Check sheet for the modelled part. Datum: model origin and axes. Units: mm. A direction names the side the tool comes from. Round coordinates to 2 decimals unless told otherwise and drop trailing zeros. Order: outer loops, then holes, each group sorted by start corner. A loop starts at its lowest first (then second) coordinate and runs counter-clockwise, first axis right, second up.
Q1. Cross-section at A-A on z = 25. Record the cut outline in (x, y).
Q2. Mould release check, pull along X, two halves, no side actions. Record for faces 1 (the flat face through (0, 5, 25)), 2 (the flat face through (45, 59, 25)), 3 (the flat face through (8.274, 8.225, 36.955)), 4 (the flat face through (51.8, 8.2, 7)): +X half, -X half, draft (parallel to the pull), parting line (faces both ways), or undercut.
Q3. Cross-section at C-C on y = 56.5. Record the cut outline in (x, z), then the cut area to 3 significant figures.
Q4. Scan lines: probe 1 along X at (y, z) = (25, 25); probe 2 along Z at (x, y) = (30, 12); probe 3 along X at (y, z) = (4, 10). Record each from-to range of solid material in increasing order.
Q5. Cross-section at D-D on z = 19. Record the cut outline in (x, y).
Q6. Set-up check for faces 5 (the cylindrical face through (12, 3, 10)), 6 (the flat face through (51.726, 8.225, 43.045)): record each of +Z, -Z, +X, -X, +Y, -Y from which the full face is reachable in a straight line by a thin tool's end or side.
Q7. Cross-section at B-B on x = 34. Record the cut outline in (y, z).
Q8. Depth check by flat-ended pin: P1, Ø24, axis at x = 22.5, y = 52, coming from the +Z side; P2, Ø3, axis at x = 29.5, z = 26, coming from the -Y side; P3, Ø2, axis at y = 91, z = 21.5, coming from the -X side; P4, Ø3.5, axis at x = 51.5, z = 8.5, coming from the +Y side. Enter the tip coordinate at first touch or a pass-through.
from build123d import *

# Parameters (mm, degrees)
SKETCH1_W           = 60
SKETCH1_H           = 50
BOSS_EXTRUDE1_DEPTH = 10
SKETCH2_R           = 2
CUT_EXTRUDE1_DEPTH  = 79.74007874
CUT_EXTRUDE2_DEPTH  = 3.6
SKETCH4_W           = 30
SKETCH4_H           = 30
BOSS_EXTRUDE2_DEPTH = 100
CUT_EXTRUDE5_START  = -30
SKETCH6_R           = 2
CUT_EXTRUDE5_DEPTH  = 30


with BuildPart() as part:
    # Sketch1 → Boss-Extrude1 (new body)
    with BuildSketch(Plane(origin=(0, 0, 0), x_dir=(1, 0, 0), z_dir=(0, 1, 0))):
        with Locations((30, -25)):
            Rectangle(SKETCH1_W, SKETCH1_H)
    extrude(amount=BOSS_EXTRUDE1_DEPTH)

    # Sketch2 → Cut-Extrude1 (cut, through all)
    with BuildSketch(Plane(origin=(0, 10, 0), x_dir=(1, 0, 0), z_dir=(0, 1, 0))):
        with Locations(Location((50, -10, 0), (0, 0, 270))):
            Circle(SKETCH2_R)
        with Locations(Location((10, -10, 0), (0, 0, 270))):
            Circle(SKETCH2_R)
        with Locations(Location((10, -40, 0), (0, 0, 270))):
            Circle(SKETCH2_R)
        with Locations(Location((50, -40, 0), (0, 0, 270))):
            Circle(SKETCH2_R)
        with Locations(Location((30, -25, 0), (0, 0, 270))):
            Circle(SKETCH2_R)
    extrude(amount=-CUT_EXTRUDE1_DEPTH, mode=Mode.SUBTRACT)

    # Sketch3 → Cut-Extrude2 (cut)
    with BuildSketch(Plane(origin=(0, 10, 0), x_dir=(1, 0, 0), z_dir=(0, 1, 0))):
        Polygon((10, -35.958548116), (6.5, -37.979274058), (6.5, -42.020725942), (10, -44.041451884), (13.5, -42.020725942), (13.5, -37.979274058), align=None)
        Polygon((50, -35.958548116), (46.5, -37.979274058), (46.5, -42.020725942), (50, -44.041451884), (53.5, -42.020725942), (53.5, -37.979274058), align=None)
        Polygon((50, -5.958548116), (46.5, -7.979274058), (46.5, -12.020725942), (50, -14.041451884), (53.5, -12.020725942), (53.5, -7.979274058), align=None)
        Polygon((10, -5.958548116), (6.5, -7.979274058), (6.5, -12.020725942), (10, -14.041451884), (13.5, -12.020725942), (13.5, -7.979274058), align=None)
    extrude(amount=-CUT_EXTRUDE2_DEPTH, mode=Mode.SUBTRACT)

    # Sketch4 → Boss-Extrude2 (add)
    with BuildSketch(Plane(origin=(0, 10, 0), x_dir=(1, 0, 0), z_dir=(0, 1, 0))):
        with Locations((30, -25)):
            Rectangle(SKETCH4_W, SKETCH4_H)
    extrude(amount=BOSS_EXTRUDE2_DEPTH)

    # Sketch6 → Cut-Extrude5 (cut)
    with BuildSketch(Plane.XZ.offset(-10).offset(CUT_EXTRUDE5_START)):
        with Locations(Location((30, 25, 0), (0, 0, 90))):
            Circle(SKETCH6_R)
    extrude(amount=CUT_EXTRUDE5_DEPTH, mode=Mode.SUBTRACT)


solid = part.part
Results found:
1. outline: (0, 0) - (28, 0) - (28, 40) - (32, 40) - (32, 0) - (60, 0) - (60, 10) - (45, 10) - (45, 110) - (15, 110) - (15, 10) - (0, 10) - close
2. face 1: -X half
2. face 2: +X half
2. face 3: undercut
2. face 4: undercut
3. outline: (15, 10) - (45, 10) - (45, 40) - (15, 40) - close
3. area: 900 mm2
4. probe 1: x = 15 to 28, 32 to 45
4. probe 2: z = 10 to 23, 27 to 40
4. probe 3: x = 0 to 8, 12 to 48, 52 to 60
5. outline: (0, 0) - (60, 0) - (60, 10) - (45, 10) - (45, 110) - (15, 110) - (15, 10) - (0, 10) - close
6. face 5: +Y, -Y
6. face 6: +Y
7. outline: (0, 0) - (10, 0) - (10, 10) - (110, 10) - (110, 40) - (10, 40) - (10, 50) - (0, 50) - close
8. P1: stops at z = 40
8. P2: stops at y = 0
8. P3: stops at x = 15
8. P4: stops at y = 10
